Geometry: see drawing. Coordinates: mm, zero at the bounding-box minimum. Coordinates: 2 decimals unless noted, no trailing zeros. Loops run counter-clockwise (first coordinate to the right, second up) from the corner with the lowest first, then second, coordinate; pieces in that order, holes last. Notation, with made-up numbers: (53.25, 1) -> (57.25, 1) arc R5 ccw to (57.25, 6) -> close; hole circle Ø2 at (3, 59). An arc over 180 degrees is marked (long way). Put each result on its own line as item: value. Start each with the question number.
1) Cut plane D-D (y = 19.75). Return the cut outline in (x, z), plus the area to 3 significant figures.
2) Cut plane C-C (z = 0.65). Return the cut outline in (x, y), plus the area to 3 significant figures.
3) Cut plane B-B (x = 24). Return the cut outline in (y, z), plus the area to 3 significant figures.
4) Contact query for a flat-ended pin moving along its axis: P1, Ø13, axis at x = 24, y = 15, coming from the -Z side. Output: stop coordinate, or through.
5) Material intervals for L1, parallel to Y at x = 42, z = 1.4; L2, parallel to Y at x = 24, z = 1.65; L3, parallel to X at y = 12.25, z = 0.9, sorted ascending.
6) Cut plane A-A (y = 15). Return the cut outline in (x, z), plus the area to 3 significant figures.
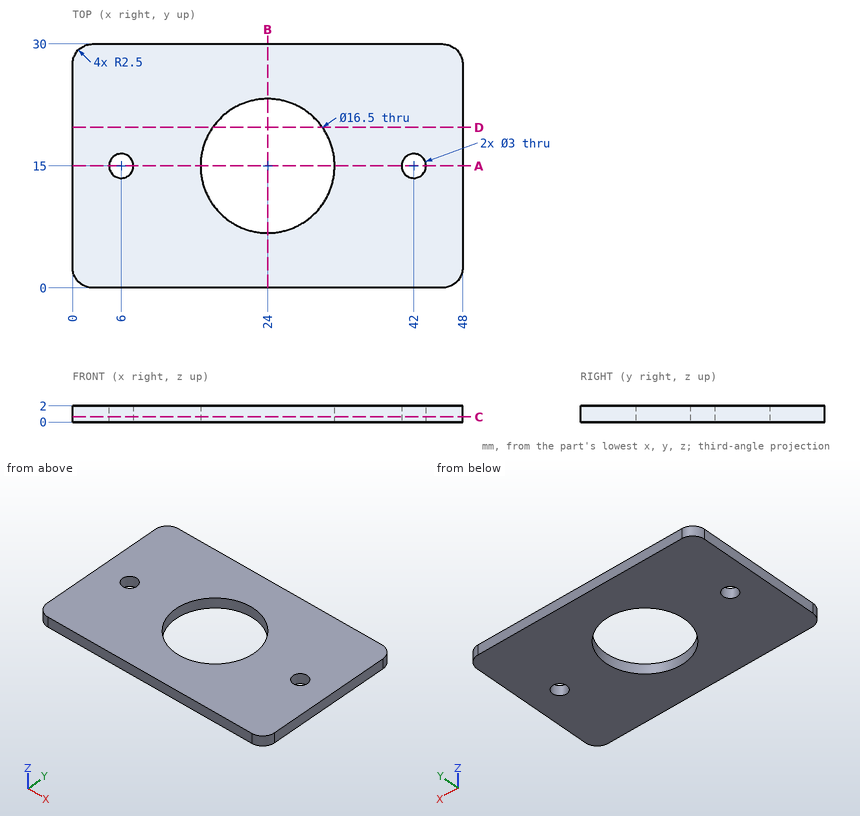
Results found:
1. outline: (0, 0) -> (17.25, 0) -> (17.25, 2) -> (0, 2) -> close; (30.75, 0) -> (48, 0) -> (48, 2) -> (30.75, 2) -> close
1. area: 69.0 mm2
2. outline: (0, 2.5) arc R2.5 ccw to (2.5, 0) -> (45.5, 0) arc R2.5 ccw to (48, 2.5) -> (48, 27.5) arc R2.5 ccw to (45.5, 30) -> (2.5, 30) arc R2.5 ccw to (0, 27.5) -> close; hole circle Ø3 at (6, 15); hole circle Ø16.5 at (24, 15); hole circle Ø3 at (42, 15)
2. area: 1,210 mm2
3. outline: (0, 0) -> (6.75, 0) -> (6.75, 2) -> (0, 2) -> close; (23.25, 0) -> (30, 0) -> (30, 2) -> (23.25, 2) -> close
3. area: 27.0 mm2
4. P1: passes through
5. L1: y = 0 to 13.5, 16.5 to 30
5. L2: y = 0 to 6.75, 23.25 to 30
5. L3: x = 0 to 16.22, 31.78 to 48
6. outline: (0, 0) -> (4.5, 0) -> (4.5, 2) -> (0, 2) -> close; (7.5, 0) -> (15.75, 0) -> (15.75, 2) -> (7.5, 2) -> close; (32.25, 0) -> (40.5, 0) -> (40.5, 2) -> (32.25, 2) -> close; (43.5, 0) -> (48, 0) -> (48, 2) -> (43.5, 2) -> close
6. area: 51.0 mm2
